Answer from the drawing. Dimensions are ordinates in mm from the lowest x, y and z of the part. A direction names the side the tool comes from. Coordinates: 2 decimals unless noted, no trailing zeros. Write each loop counter-clockwise with the first axis right and the second up, starting at its lowest first coordinate (ties: lowest second). Pieces come first, ordered by that corner, then holes. Notation, with made-up numbers: (-39, -1.75) -> (-6, -1.75) arc R15 cw to (-6, 12.25) -> close; hole circle Ø9 at (73, -17). An arc over 180 degrees is marked (long way). One line per item, written item: value. Start each with the question number.
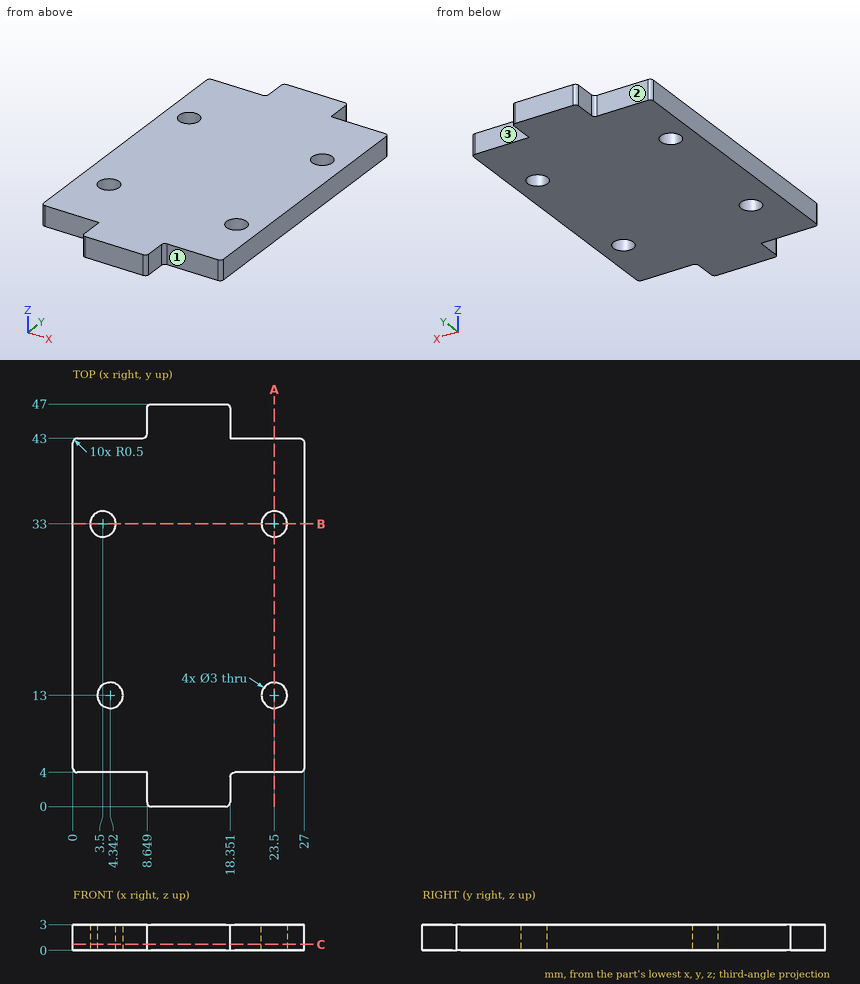
1. A tool of negligible diameter and unlimited length cuts with its end or side. For the marked faces 1, 2 and 3, from which of +Z, -Z, +X, -X, +Y, -Y can it reach the whole face along a straight path? Write none if from no direction.
2. A cutting plane is placed at C-C on z = 0.7. Give the vertices of the cut face in (x, y).
3. Find the intervals of material crossed by probe 1 along Y at (x, z) = (23.5, 0.65); probe 2 along X at (y, z) = (33.5, 0.5) (1 decimal); probe 3 along Y at (x, z) = (22.25, 2.95), in increasing order. Write a range as from..to.
4. Given pin 1 (0.9 mm diameter, centred on y = 45.5, z = 1, fed in from +X), flat-ended and moving along its own axis, determine where the tip first touches the part or whether it passes through.
5. A cutting plane is placed at B-B on y = 33. Give the vertices of the cut face in (x, z).
6. A cutting plane is placed at A-A on x = 23.5. Give the vertices of the cut face in (y, z).
Derived:
1. face 1: +Z, -Z, +X, -Y
1. face 2: +Z, -Z, -X, +Y
1. face 3: +Z, -Z, +X, +Y
2. outline: (0, 4.5) arc R0.5 ccw to (0.5, 4) -> (8.65, 4) -> (8.65, 0.5) arc R0.5 ccw to (9.15, 0) -> (17.85, 0) arc R0.5 ccw to (18.35, 0.5) -> (18.35, 3.5) arc R0.5 cw to (18.85, 4) -> (26.5, 4) arc R0.5 ccw to (27, 4.5) -> (27, 42.5) arc R0.5 ccw to (26.5, 43) -> (18.35, 43) -> (18.35, 46.5) arc R0.5 ccw to (17.85, 47) -> (9.15, 47) arc R0.5 ccw to (8.65, 46.5) -> (8.65, 43.5) arc R0.5 cw to (8.15, 43) -> (0.5, 43) arc R0.5 ccw to (0, 42.5) -> close; hole circle Ø3 at (3.5, 33); hole circle Ø3 at (4.34, 13); hole circle Ø3 at (23.5, 13); hole circle Ø3 at (23.5, 33)
3. probe 1: y = 4..11.5, 14.5..31.5, 34.5..43
3. probe 2: x = 0..2.1, 4.9..22.1, 24.9..27
3. probe 3: y = 4..12.17, 13.83..32.17, 33.83..43
4. pin 1: stops at x = 18.35
5. outline: (0, 0) -> (2, 0) -> (2, 3) -> (0, 3) -> close; (5, 0) -> (22, 0) -> (22, 3) -> (5, 3) -> close; (25, 0) -> (27, 0) -> (27, 3) -> (25, 3) -> close
6. outline: (4, 0) -> (11.5, 0) -> (11.5, 3) -> (4, 3) -> close; (14.5, 0) -> (31.5, 0) -> (31.5, 3) -> (14.5, 3) -> close; (34.5, 0) -> (43, 0) -> (43, 3) -> (34.5, 3) -> close
